```python
from build123d import *

# Parameters (mm, degrees)
BOSS_EXTRUDE1_DEPTH = 1.524


with BuildPart() as part:
    # Sketch1 → Boss-Extrude1 (new body)
    with BuildSketch(Plane.XY):
        with BuildLine():
            Line((216.672701746, -0.007446462), (216.672701746, -2.547446462))
            Line((216.672701746, -2.547446462), (202.922883793, -2.527561419))
            ThreePointArc((202.922883793, -2.527561419), (213.740389033, -12.255488314), (228.152940708, -14.237743463))
            ThreePointArc((228.152940708, -14.237743463), (229.539309592, -15.004139991), (230.201920973, -16.443003598))
            ThreePointArc((230.201920973, -16.443003598), (231.794065838, -22.769182164), (234.983138477, -28.459988454))
            ThreePointArc((234.983138477, -28.459988454), (228.404400606, -42.301387702), (232.479424339, -57.074955542))
            ThreePointArc((232.479424339, -57.074955542), (228.088258842, -58.913193865), (224.685678773, -62.242443545))
            ThreePointArc((224.685678773, -62.242443545), (223.318434752, -63.974353777), (221.232380668, -64.693553069))
            ThreePointArc((221.232380668, -64.693553069), (200.556241101, -64.829244423), (180.56810467, -59.538161211))
            ThreePointArc((180.56810467, -59.538161211), (177.088182276, -59.862533625), (175.243626571, -62.831151415))
            ThreePointArc((175.243626571, -62.831151415), (168.436022627, -67.194555572), (165.179908551, -74.595939794))
            ThreePointArc((165.179908551, -74.595939794), (180.56810467, -71.491688256), (196.088301261, -73.848901695))
            ThreePointArc((196.088301261, -73.848901695), (201.561550117, -74.595878453), (207.085536659, -74.595939794))
            ThreePointArc((207.085536659, -74.595939794), (218.25265241, -73.536219791), (229.434140266, -74.431658236))
            ThreePointArc((229.434140266, -74.431658236), (232.368160186, -73.324137561), (231.528773962, -70.302464895))
            ThreePointArc((231.528773962, -70.302464895), (230.749723909, -69.684443769), (230.004496974, -69.026032112))
            Line((230.004496974, -69.026032112), (199.761798891, -69.011393679))
            Line((199.761798891, -69.011393679), (199.761798891, -67.487393679))
            Line((199.761798891, -67.487393679), (234.591320158, -67.44538381))
            ThreePointArc((234.591320158, -67.44538381), (235.566450517, -67.25102819), (236.542114519, -67.059369434))
            Line((236.542114519, -67.059369434), (241.754501837, -33.540074699))
            Line((241.754501837, -33.540074699), (243.260404343, -33.774248693))
            Line((243.260404343, -33.774248693), (238.132067507, -66.75304007))
            ThreePointArc((238.132067507, -66.75304007), (239.89605254, -66.421852491), (241.661668499, -66.099472755))
            ThreePointArc((241.661668499, -66.099472755), (245.789044159, -63.002771973), (246.435787058, -57.883542618))
            ThreePointArc((246.435787058, -57.883542618), (245.449591498, -44.052865168), (252.944866234, -32.387485746))
            ThreePointArc((252.944866234, -32.387485746), (253.618048182, -31.554800294), (253.888271711, -30.518693039))
            ThreePointArc((253.888271711, -30.518693039), (254.1727268, -26.934998032), (254.717509197, -23.381549463))
            ThreePointArc((254.717509197, -23.381549463), (254.684120067, -22.279090661), (254.186569515, -21.294726048))
            ThreePointArc((254.186569515, -21.294726048), (254.359804188, -12.854167351), (257.874930037, -5.178430798))
            ThreePointArc((257.874930037, -5.178430798), (258.196394426, -3.928637169), (257.862228141, -2.682179643))
            ThreePointArc((257.862228141, -2.682179643), (241.364921289, 10.401189736), (220.392134228, 12.266100085))
            ThreePointArc((220.392134228, 12.266100085), (220.341626443, 12.255208572), (220.291350651, 12.243291934))
            Line((220.291350651, 12.243291934), (205.161370791, 8.494168867))
            ThreePointArc((205.161370791, 8.494168867), (203.913862316, 7.760159754), (203.269847057, 6.463899318))
            Line((203.269847057, 6.463899318), (202.1481549, 0.013558997))
            Line((202.1481549, 0.013558997), (216.672701746, -0.007446462))
        make_face()
    extrude(amount=BOSS_EXTRUDE1_DEPTH)


solid = part.part
```
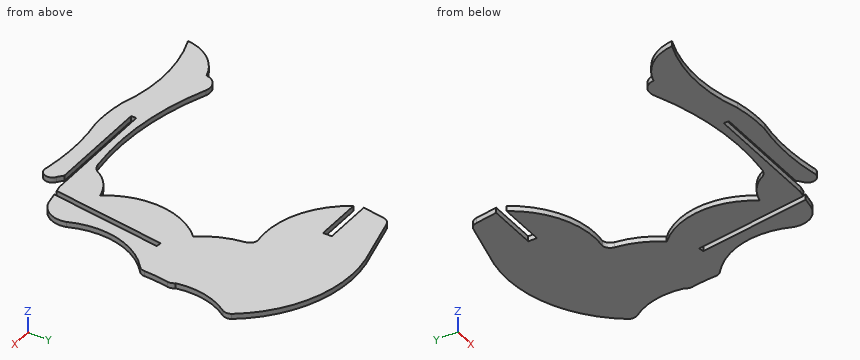
Part model, mm, in its own coordinate system. Give positions to 0.01 mm unless a question says otherwise; leave off trailing zeros. Write each loop counter-clockwise with the first axis right and the second up, starting at its lowest first coordinate (ties: lowest second). Pieces come first, ordered by that corner, then holes. Notation, with made-up numbers: M 56.5,2.25 L 71.5,2.25 A34 ccw 71.5,36.25 Z; hole C 75.5,71.25 d9. An arc over 180 degrees is marked long. Use CSV: the item, a comma, the result in double quotes.
Item 1: Slice it at D-D on y = -10.5. Write the cut outline in (x, z).
Taken from the geometry:
outline,"M 210.58,0 L 255.05,0 L 255.05,1.52 L 210.58,1.52 Z"
Item 2: Slice it at C-C on x = 249. Write the cut outline in (y, z).
Taken from the geometry:
outline,"M -36.52,0 L 6.25,0 L 6.25,1.52 L -36.52,1.52 Z"
Item 3: Slice it at A-A on x = 211.5. Write the cut outline in (y, z), plus the area to 3 significant figures.
Taken from the geometry:
outline,"M -73.94,0 L -69.02,0 L -69.02,1.52 L -73.94,1.52 Z; M -67.47,0 L -65.44,0 L -65.44,1.52 L -67.47,1.52 Z; M -11.07,0 L -2.54,0 L -2.54,1.52 L -11.07,1.52 Z; M 0,0 L 10.06,0 L 10.06,1.52 L 0,1.52 Z"
area,"38.9 mm²"
Item 4: Slice it at B-B on y = -44.5. Write the cut outline in (x, z), plus the area to 3 significant figures.
Taken from the geometry:
outline,"M 228.32,0 L 240.05,0 L 240.05,1.52 L 228.32,1.52 Z; M 241.59,0 L 245.34,0 L 245.34,1.52 L 241.59,1.52 Z"
area,"23.6 mm²"
Item 5: Drill centre lines: probe 1 along Y at (x, z) = (217.5, 1.2); probe 2 along Y at (x, z) = (226, 0.7); probe 3 along Y at (x, z) = (207.5, 1.1). Where is each one in solid material? Low to high.
Taken from the geometry:
probe 1,"y = -73.55 to -69.02, -67.47 to -65.13, -13.64 to 11.55"
probe 2,"y = -73.95 to -69.02, -67.46 to -60.65, -14.49 to 12.97"
probe 3,"y = -74.52 to -69.02, -67.48 to -65.4, -8.11 to -2.53, 0.01 to 9.07"
